from build123d import *

# Parameters (mm, degrees)
SKETCH1_R           = 1.5
BOSS_EXTRUDE1_DEPTH = 3


with BuildPart() as part:
    # Sketch1 → Boss-Extrude1 (new body)
    with BuildSketch(Plane(origin=(0, 0, 0), x_dir=(1, 0, 0), z_dir=(0, 1, 0))):
        with BuildLine():
            Line((65, 15.5), (58.5, 15.5))
            ThreePointArc((58.5, 15.5), (57.085786438, 14.914213562), (56.5, 13.5))
            Line((56.5, 13.5), (56.5, 7.5))
            ThreePointArc((56.5, 7.5), (55.914213562, 6.085786438), (54.5, 5.5))
            Line((54.5, 5.5), (47.5, 5.5))
            ThreePointArc((47.5, 5.5), (46.085786438, 6.085786438), (45.5, 7.5))
            Line((45.5, 7.5), (45.5, 13.5))
            ThreePointArc((45.5, 13.5), (44.914213562, 14.914213562), (43.5, 15.5))
            Line((43.5, 15.5), (41.5, 15.5))
            ThreePointArc((41.5, 15.5), (40.085786438, 14.914213562), (39.5, 13.5))
            Line((39.5, 13.5), (39.5, 7.5))
            ThreePointArc((39.5, 7.5), (38.914213562, 6.085786438), (37.5, 5.5))
            Line((37.5, 5.5), (30.5, 5.5))
            ThreePointArc((30.5, 5.5), (29.085786438, 6.085786438), (28.5, 7.5))
            Line((28.5, 7.5), (28.5, 13.5))
            ThreePointArc((28.5, 13.5), (27.914213562, 14.914213562), (26.5, 15.5))
            Line((26.5, 15.5), (24.5, 15.5))
            ThreePointArc((24.5, 15.5), (23.085786438, 14.914213562), (22.5, 13.5))
            Line((22.5, 13.5), (22.5, 7.5))
            ThreePointArc((22.5, 7.5), (21.914213562, 6.085786438), (20.5, 5.5))
            Line((20.5, 5.5), (13.5, 5.5))
            ThreePointArc((13.5, 5.5), (12.085786438, 6.085786438), (11.5, 7.5))
            Line((11.5, 7.5), (11.5, 13.5))
            ThreePointArc((11.5, 13.5), (10.914213562, 14.914213562), (9.5, 15.5))
            Line((9.5, 15.5), (7.5, 15.5))
            ThreePointArc((7.5, 15.5), (6.085786438, 14.914213562), (5.5, 13.5))
            Line((5.5, 13.5), (5.5, 7.5))
            ThreePointArc((5.5, 7.5), (4.914213562, 6.085786438), (3.5, 5.5))
            Line((3.5, 5.5), (-3.5, 5.5))
            ThreePointArc((-3.5, 5.5), (-4.914213562, 6.085786438), (-5.5, 7.5))
            Line((-5.5, 7.5), (-5.5, 13.5))
            ThreePointArc((-5.5, 13.5), (-6.085786438, 14.914213562), (-7.5, 15.5))
            Line((-7.5, 15.5), (-9.5, 15.5))
            ThreePointArc((-9.5, 15.5), (-10.914213562, 14.914213562), (-11.5, 13.5))
            Line((-11.5, 13.5), (-11.5, 7.5))
            ThreePointArc((-11.5, 7.5), (-12.085786438, 6.085786438), (-13.5, 5.5))
            Line((-13.5, 5.5), (-20.5, 5.5))
            ThreePointArc((-20.5, 5.5), (-21.914213562, 6.085786438), (-22.5, 7.5))
            Line((-22.5, 7.5), (-22.5, 13.5))
            ThreePointArc((-22.5, 13.5), (-23.085786438, 14.914213562), (-24.5, 15.5))
            Line((-24.5, 15.5), (-26.5, 15.5))
            ThreePointArc((-26.5, 15.5), (-27.914213562, 14.914213562), (-28.5, 13.5))
            Line((-28.5, 13.5), (-28.5, 7.5))
            ThreePointArc((-28.5, 7.5), (-29.085786438, 6.085786438), (-30.5, 5.5))
            Line((-30.5, 5.5), (-37.5, 5.5))
            ThreePointArc((-37.5, 5.5), (-38.914213562, 6.085786438), (-39.5, 7.5))
            Line((-39.5, 7.5), (-39.5, 13.5))
            ThreePointArc((-39.5, 13.5), (-40.085786438, 14.914213562), (-41.5, 15.5))
            Line((-41.5, 15.5), (-43.5, 15.5))
            ThreePointArc((-43.5, 15.5), (-44.914213562, 14.914213562), (-45.5, 13.5))
            Line((-45.5, 13.5), (-45.5, 7.5))
            ThreePointArc((-45.5, 7.5), (-46.085786438, 6.085786438), (-47.5, 5.5))
            Line((-47.5, 5.5), (-54.5, 5.5))
            ThreePointArc((-54.5, 5.5), (-55.914213562, 6.085786438), (-56.5, 7.5))
            Line((-56.5, 7.5), (-56.5, 13.5))
            ThreePointArc((-56.5, 13.5), (-57.085786438, 14.914213562), (-58.5, 15.5))
            Line((-58.5, 15.5), (-65, 15.5))
            ThreePointArc((-65, 15.5), (-68.535533906, 14.035533906), (-70, 10.5))
            Line((-70, 10.5), (-70, -10.5))
            ThreePointArc((-70, -10.5), (-68.535533906, -14.035533906), (-65, -15.5))
            Line((-65, -15.5), (65, -15.5))
            ThreePointArc((65, -15.5), (68.535533906, -14.035533906), (70, -10.5))
            Line((70, -10.5), (70, 10.5))
            ThreePointArc((70, 10.5), (68.535533906, 14.035533906), (65, 15.5))
        make_face()
        with Locations((-65.5, 0)):
            Circle(SKETCH1_R, mode=Mode.SUBTRACT)
        with Locations((65.5, 0)):
            Circle(SKETCH1_R, mode=Mode.SUBTRACT)
        with Locations((-51, -8.5)):
            Circle(SKETCH1_R, mode=Mode.SUBTRACT)
        with Locations((-34, -8.5)):
            Circle(SKETCH1_R, mode=Mode.SUBTRACT)
        with Locations((-17, -8.5)):
            Circle(SKETCH1_R, mode=Mode.SUBTRACT)
        with Locations((0, -8.5)):
            Circle(SKETCH1_R, mode=Mode.SUBTRACT)
        with Locations((17, -8.5)):
            Circle(SKETCH1_R, mode=Mode.SUBTRACT)
        with Locations((34, -8.5)):
            Circle(SKETCH1_R, mode=Mode.SUBTRACT)
        with Locations((51, -8.5)):
            Circle(SKETCH1_R, mode=Mode.SUBTRACT)
    extrude(amount=BOSS_EXTRUDE1_DEPTH)


solid = part.part
Can you work these out from the model? Positions are in its coordinate system, mm. A direction names the side the tool comes from. Give positions to 0.01 mm unless a question says otherwise; leave off trailing zeros. Order: outer loops, then holes, each group sorted by start corner. A loop starts at its lowest first (then second) coordinate and runs counter-clockwise, first axis right, second up. Notation, with made-up numbers: M -35,-25 L -23,-25 A28 ccw -23,5 Z; hole C 58.25,71.25 d2. An arc over 180 degrees is marked long. One line per question, with ' | ' between items.
Item 1: I'm going to push flat-ended pins straight in: pin 1 Ø1 at (x, y) = (36, 2.5) entering from -Z; pin 2 Ø2.5 at (x, z) = (-17, 8.5) entering from -Y. Where does each tip first touch, or does it pass through?
Answer block:
pin 1: stops at z = -5.5 | pin 2: passes through
Item 2: Please list where these lines run through material, in increasing order: L1, parallel to Z at x = 17, y = 1.65; L2, parallel to Z at x = 32, y = 0.5; L3, parallel to Z at x = -33, y = 0.9.
Answer block:
L1: z = -5.5 to 7, 10 to 15.5 | L2: z = -5.5 to 15.5 | L3: z = -5.5 to 7.38, 9.62 to 15.5
Item 3: For faces 5 (the face through (67, 1, 0)), 6 (the face through (-28.5, 1, -11)), which set-ups out of +Z, -Z, +X, -X, +Y, -Y let a thin tool reach every point of the face, with its end or its side?
Answer block:
face 5: +Y, -Y | face 6: -Z, +Y, -Y
Item 4: We'd pull the mould along X, two halves only. Please class faces 1 (the face through (-1, 0, 3)), 2 (the face through (-35.2, 1.5, 9.4)), 3 (the face through (-68.57, 1.48, 14)), 4 (the face through (70, 1, 0)): released by +X, released by -X, zero draft, split by the parting line, or undercut.
Answer block:
face 1: zero draft | face 2: undercut | face 3: released by -X | face 4: released by +X
Item 5: Suppose I cut it at B-B, the plane x = -17. Write out the boundary of the cut face in (y, z).
Answer block:
outline: M 0,-5.5 L 3,-5.5 L 3,7 L 0,7 Z; M 0,10 L 3,10 L 3,15.5 L 0,15.5 Z
Item 6: Suppose I cut it at A-A, the plane z = 0. Write out the boundary of the cut face in (x, y), then the cut area to 3 significant figures.
Answer block:
outline: M -70,0 L -67,0 L -67,3 L -70,3 Z; M -64,0 L 64,0 L 64,3 L -64,3 Z; M 67,0 L 70,0 L 70,3 L 67,3 Z | area: 402 mm2
Item 7: Suppose I cut it at C-C, the plane y = 2.45. Give the number of separate pieces and of enclosed holes in the cut face, then the cut area to 3 significant figures.
Answer block:
separate pieces: 1 | enclosed holes: 9 | area: 3,480 mm2
